```python
from build123d import *

# Parameters (mm, degrees)
BOSS_EXTRUDE1_DEPTH = 3.175


with BuildPart() as part:
    # Sketch1 → Boss-Extrude1 (new body)
    with BuildSketch(Plane.XY):
        with BuildLine():
            Line((-50.564988155, 9.325788887), (-61.025093708, 9.325788887))
            Line((-61.025093708, 9.325788887), (-61.025093708, 12.500788887))
            Line((-61.025093708, 12.500788887), (-80.363597484, 12.500788887))
            Line((-80.363597484, 12.500788887), (-80.363597484, 9.325788887))
            Line((-80.363597484, 9.325788887), (-90.564988155, 9.325788887))
            add(Edge.make_bspline(
                [(-50.564988155, -20.674211113), (-78.351175561, -18.870925546), (-90.564988155, 9.325788887)],
                knots=[0, 0, 0, 1, 1, 1], degree=2))
            Line((-50.564988155, -20.674211113), (-50.564988155, -6.674211113))
            Line((-50.564988155, -6.674211113), (-46.911258203, -6.674211113))
            Line((-46.911258203, -6.674211113), (-46.911258203, 3.325788887))
            Line((-46.911258203, 3.325788887), (-50.564988155, 3.325788887))
            Line((-50.564988155, 3.325788887), (-50.564988155, 9.325788887))
        make_face()
    extrude(amount=BOSS_EXTRUDE1_DEPTH)


solid = part.part
```
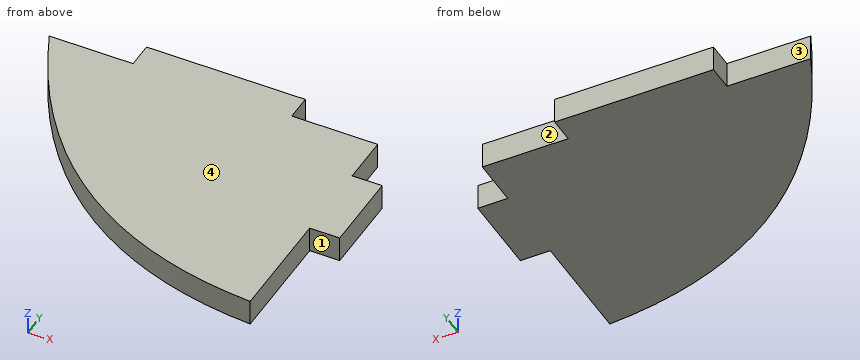
For this review, take the finished solid that the model builds, in its own axes (mm). Face numbers are marked on the shaded views. A direction names the side the tool comes from. Round coordinates to 2 decimals unless told otherwise and drop trailing zeros. Write each loop counter-clockwise with the first axis right and the second up, starting at its lowest first coordinate (ties: lowest second). Pieces come first, ordered by that corner, then holes. Notation, with made-up numbers: (79.5, 49) -> (96.5, 49) arc R25 cw to (96.5, 70) -> close; hole circle Ø11 at (8.5, 81.5). An arc over 180 degrees is marked (long way). Use one line per item in the form item = value.
Q1. To check wall thickness, follow probe 1 along Y at (x, z) = (-48.5, 1.6); probe 2 along Y at (x, z) = (-85.5, 2.3); probe 3 along X at (y, z) = (1, 0.4). State the ranges of each line that lie inside material, in increasing order. Write a range as from..to.
Resolved:
probe_1 = -6.67..3.33
probe_2 = -0.22..9.33
probe_3 = -86.27..-46.91
Q2. Consider section A-A (y = 10). State the section outline as (x, z) points (3 decimals).
Resolved:
outline = (-80.364, 0) -> (-61.025, 0) -> (-61.025, 3.175) -> (-80.364, 3.175) -> close
Q3. Clearance check with flat-ended pins moving along their axes: pin 1 Ø1.6 at (y, z) = (11, 1) entering from -X; pin 2 Ø1.6 at (y, z) = (-10.5, 1.5) entering from +X (3 decimals); pin 3 Ø1.6 at (x, z) = (-48, 2.5) entering from -Y. State where each tip first meets the part, or that it passes through.
Resolved:
pin_1 = -80.36
pin_2 = -50.565
pin_3 = -6.67
Q4. Machinability: for the marked faces 1, 2, 3 and 4, which of the approach directions +Z, -Z, +X, -X, +Y, -Y give a long, thin tool a straight path to every point of the face, cutting with its end or side? Answer none if there is none.
Resolved:
face_1 = +Z, -Z, +X, -Y
face_2 = +Z, -Z, +X, +Y
face_3 = +Z, -Z, -X, +Y
face_4 = +Z, +X, -X, +Y, -Y
